Check sheet for the modelled part. Datum: model origin and axes. Units: mm. A direction names the side the tool comes from. Give positions to 0.01 mm unless a question says otherwise; leave off trailing zeros. Write each loop counter-clockwise with the first axis right and the second up, starting at its lowest first coordinate (ties: lowest second). Pieces come first, ordered by that corner, then holes. Notation, with made-up numbers: (44, -5.5) -> (96, -5.5) arc R5 ccw to (96, 1.5) -> close; hole circle Ø7 at (76, -3.5). An arc over 180 degrees is marked (long way). Use a Markdown table: item, result. Add a question column.
1. Release check for a two-part mould opening along Z. For faces 3 (the flat face through (0, 2, -27.4)), 4 (the flat face through (18, 2, 0)), 5 (the flat face through (0, 2, 22.4)), 6 (the flat face through (-27.4, 2, 0)) record: released by +Z, released by -Z, zero draft, split by the parting line, or undercut.
2. Cross-section at D-D (z = -10.7). Enter the section's corners in (x, y), then the cut area to 3 significant figures.
3. Gauge pin test, flat end, axial feed: P1, Ø3, axis at x = 10.7, z = 10.7, coming from the -Y side. Record the tip position at first contact, or that the pin passes through.
4. Cross-section at C-C (y = 2.85). Count the separate pieces of the cut face and the enclosed holes in it, then the cut area to 3 significant figures.
5. Cross-section at A-A (x = -7). Enter the section's corners in (y, z), then the cut area to 3 significant figures.
6. Set-up check for faces 1 (the flat face through (27.4, 2, 0)), 2 (the flat face through (-20, 2, -13)): record each of +Z, -Z, +X, -X, +Y, -Y from which the full face is reachable in a straight line by a thin tool's end or side.
7. Cross-section at B-B (x = 0). Enter the section's corners in (y, z), then the cut area to 3 significant figures.
8. Scan lines: probe 1 along X at (y, z) = (2.9, 21.4); probe 2 along Z at (x, y) = (0, 1.4); probe 3 along X at (y, z) = (1.1, -10.7). Record each from-to range of solid material in increasing order. Write a range as [from, to].
from build123d import *

# Parameters (mm, degrees)
SKETCH_1_W          = 54.8
SKETCH_1_H          = 54.8
SKETCH_1_R          = 4.1
SKETCH_1_R_2        = 1.6
EXTRUDE_1_DEPTH     = 4.4
FILLET_1_R          = 6
SKETCH_2_R          = 1.6
CUT_EXTRUDE_1_DEPTH = 10


with BuildPart() as part:
    # 草图1 → 凸台-拉伸1 (new body)
    with BuildSketch(Plane(origin=(0, 0, 0), x_dir=(1, 0, 0), z_dir=(0, 1, 0))):
        Rectangle(SKETCH_1_W, SKETCH_1_H)
        Circle(SKETCH_1_R, mode=Mode.SUBTRACT)
        with Locations((21.4, 21.4)):
            Circle(SKETCH_1_R_2, mode=Mode.SUBTRACT)
        with Locations((21.4, -21.4)):
            Circle(SKETCH_1_R_2, mode=Mode.SUBTRACT)
        with Locations((-21.4, -21.4)):
            Circle(SKETCH_1_R_2, mode=Mode.SUBTRACT)
        with Locations((-21.4, 21.4)):
            Circle(SKETCH_1_R_2, mode=Mode.SUBTRACT)
        Polygon((18, -5), (18, 5), (18, 13), (22.4, 13), (22.4, 5), (22.4, -5), (22.4, -13), (18, -13), align=None, mode=Mode.SUBTRACT)
        Polygon((-5, 18), (-13, 18), (-13, 22.4), (-5, 22.4), (5, 22.4), (13, 22.4), (13, 18), (5, 18), align=None, mode=Mode.SUBTRACT)
        Polygon((5, -18), (13, -18), (13, -22.4), (5, -22.4), (-5, -22.4), (-13, -22.4), (-13, -18), (-5, -18), align=None, mode=Mode.SUBTRACT)
        Polygon((-18, 5), (-18, -5), (-18, -13), (-22.4, -13), (-22.4, -5), (-22.4, 5), (-22.4, 13), (-18, 13), align=None, mode=Mode.SUBTRACT)
    extrude(amount=EXTRUDE_1_DEPTH)

    # 圆角1
    fillet_1_edges = [part.edges().sort_by_distance(p)[0] for p in [
        (27.4, 2.2, 27.4),
        (-27.4, 2.2, 27.4),
        (-27.4, 2.2, -27.4),
        (27.4, 2.2, -27.4),
    ]]
    fillet(fillet_1_edges, radius=FILLET_1_R)

    # 草图2 → 切除-拉伸1 (cut)
    with BuildSketch(Plane(origin=(0, 4.4, 0), x_dir=(1, 0, 0), z_dir=(0, 1, 0))):
        with Locations((10.7, 10.7)):
            Circle(SKETCH_2_R)
        with Locations((10.7, -10.7)):
            Circle(SKETCH_2_R)
        with Locations((-10.7, -10.7)):
            Circle(SKETCH_2_R)
        with Locations((-10.7, 10.7)):
            Circle(SKETCH_2_R)
    extrude(amount=-CUT_EXTRUDE_1_DEPTH, mode=Mode.SUBTRACT)


solid = part.part
Worked answers:
| question | item | result |
|---|---|---|
| 1 | face 3 | released by -Z |
| 1 | face 4 | undercut |
| 1 | face 5 | undercut |
| 1 | face 6 | zero draft |
| 2 | outline | (-27.4, 0) -> (-22.4, 0) -> (-22.4, 4.4) -> (-27.4, 4.4) -> close; (-18, 0) -> (-12.3, 0) -> (-12.3, 4.4) -> (-18, 4.4) -> close; (-9.1, 0) -> (9.1, 0) -> (9.1, 4.4) -> (-9.1, 4.4) -> close; (12.3, 0) -> (18, 0) -> (18, 4.4) -> (12.3, 4.4) -> close; (22.4, 0) -> (27.4, 0) -> (27.4, 4.4) -> (22.4, 4.4) -> close |
| 2 | area | 174 mm² |
| 3 | P1 | passes through |
| 4 | separate pieces | 1 |
| 4 | enclosed holes | 13 |
| 4 | area | 2,400 mm² |
| 5 | outline | (0, -27.4) -> (4.4, -27.4) -> (4.4, -22.4) -> (0, -22.4) -> close; (0, -18) -> (4.4, -18) -> (4.4, 18) -> (0, 18) -> close; (0, 22.4) -> (4.4, 22.4) -> (4.4, 27.4) -> (0, 27.4) -> close |
| 5 | area | 202 mm² |
| 6 | face 1 | +Z, -Z, +X, +Y, -Y |
| 6 | face 2 | +Y, -Y |
| 7 | outline | (0, -27.4) -> (4.4, -27.4) -> (4.4, -22.4) -> (0, -22.4) -> close; (0, -18) -> (4.4, -18) -> (4.4, -4.1) -> (0, -4.1) -> close; (0, 4.1) -> (4.4, 4.1) -> (4.4, 18) -> (0, 18) -> close; (0, 22.4) -> (4.4, 22.4) -> (4.4, 27.4) -> (0, 27.4) -> close |
| 7 | area | 166 mm² |
| 8 | probe 1 | x = [-27.4, -23], [-19.8, -13], [13, 19.8], [23, 27.4] |
| 8 | probe 2 | z = [-27.4, -22.4], [-18, -4.1], [4.1, 18], [22.4, 27.4] |
| 8 | probe 3 | x = [-27.4, -22.4], [-18, -12.3], [-9.1, 9.1], [12.3, 18], [22.4, 27.4] |
